Input: part model. Units: mm. Frame: model coordinates. Face numbers are marked on the shaded views. A direction names the side the tool comes from. Give positions to 0.01 mm unless a question says otherwise; leave off trailing zeros. Loops run counter-clockwise (first coordinate to the right, second up) from the corner with the lowest first, then second, coordinate; pieces in that order, holes last. Notation, with made-up numbers: (66.25, -14.75) -> (74.25, -14.75) arc R14 cw to (74.25, 8.25) -> close; hole circle Ø2 at (7, 1). An arc over 180 degrees is marked (long way). Answer as a JSON object with one key per item and string values. Group by question number.
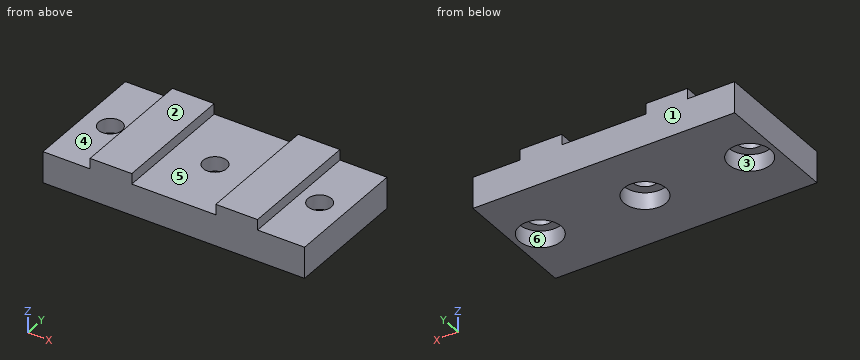
```python
from build123d import *

# Parameters (mm, degrees)
SKETCH1_W          = 39.6748
SKETCH1_H          = 19.05
EXTRUDE1_DEPTH     = 6.35
SKETCH2_W          = 7.1374
SKETCH2_H          = 1.6002
SKETCH2_W_2        = 12.7508
CUT_EXTRUDE1_DEPTH = 20.05
HOLE1_D            = 3.556
HOLE1_CBORE_D      = 6.35
HOLE1_CBORE_DEPTH  = 2.54


with BuildPart() as part:
    # Sketch1 → Extrude1 (new body)
    with BuildSketch(Plane.XY):
        with Locations((19.8374, 9.525)):
            Rectangle(SKETCH1_W, SKETCH1_H)
    extrude(amount=EXTRUDE1_DEPTH)

    # Sketch2 → Cut-Extrude1 (cut, through all)
    with BuildSketch(Plane.XZ):
        with Locations((3.5687, 5.5499)):
            Rectangle(SKETCH2_W, SKETCH2_H)
        with Locations((19.8374, 5.5499)):
            Rectangle(SKETCH2_W_2, SKETCH2_H)
        with Locations((36.1061, 5.5499)):
            Rectangle(SKETCH2_W, SKETCH2_H)
    extrude(amount=-CUT_EXTRUDE1_DEPTH, mode=Mode.SUBTRACT)

    # Hole1 (through all)
    with Locations(Plane(origin=(0, 0, 0), x_dir=(-1, 0, 0), z_dir=(0, 0, -1))):
        with Locations((-3.9624, 9.525), (-19.8374, 9.525), (-35.7124, 9.525)):
            CounterBoreHole(HOLE1_D / 2, HOLE1_CBORE_D / 2, HOLE1_CBORE_DEPTH)


solid = part.part
```
Q1. Ray query, probe 1 along X at (y, z) = (8.5, 3.75); probe 2 along Z at (x, y) = (26, 11.75); probe 3 along Y at (x, z) = (4, 0.5). Return the intervals inside material, ascending.
Q2. Section B-B on z = 4.25. Return the cut outline in (x, y) (3 decimals), then the cut area to 3 significant figures.
Q3. Section A-A on x = 35.5. Return the cut outline in (y, z), then the cut area to 3 significant figures.
Q4. Pull-direction query (Y, two-part tool) for the marked faces 1, 2 and 3; classes: +Y half, -Y half, draft (parallel to the pull), parting line (faces both ways), or undercut.
Q5. Section C-C on y = 2.75. Return the cut outline in (x, z), then the cut area to 3 significant figures.
Q6. Section D-D on x = 19.5. Return the cut outline in (y, z), then the cut area to 3 significant figures.
Q7. Set-up query: the marked faces 4, 5 and 6. Return all of +Z, -Z, +X, -X, +Y, -Y with unobstructed straight access to the full face (end or side cutting, diameter ignored); none if empty.
Q8. Pin query (flat end, axial travel): pin 1 Ø0.5 at (y, z) = (11.5, 5.5) entering from +X; pin 2 Ø5 at (x, y) = (18.5, 8.5) entering from -Z; pin 3 Ø4.5 at (x, y) = (3.96, 9.52) entering from +Z; pin 4 Ø3 at (x, y) = (19.84, 9.52) entering from +Z. Return the tip coordinate at first contact, or that it passes through.
Numbers:
{
 "1": {"probe 1": "x = 0 to 2.51, 5.42 to 18.38, 21.29 to 34.26, 37.17 to 39.67", "probe 2": "z = 0 to 4.75", "probe 3": "y = 0 to 6.35, 12.7 to 19.05"},
 "2": {"outline": "(0, 0) -> (39.675, 0) -> (39.675, 19.05) -> (0, 19.05) -> close; hole circle Ø3.556 at (3.962, 9.525); hole circle Ø3.556 at (19.837, 9.525); hole circle Ø3.556 at (35.712, 9.525)", "area": "726 mm²"},
 "3": {"outline": "(0, 0) -> (6.36, 0) -> (6.36, 2.54) -> (7.76, 2.54) -> (7.76, 4.75) -> (0, 4.75) -> close; (11.29, 2.54) -> (12.69, 2.54) -> (12.69, 0) -> (19.05, 0) -> (19.05, 4.75) -> (11.29, 4.75) -> close", "area": "66.6 mm²"},
 "4": {"face 1": "+Y half", "face 2": "draft", "face 3": "undercut"},
 "5": {"outline": "(0, 0) -> (39.67, 0) -> (39.67, 4.75) -> (32.54, 4.75) -> (32.54, 6.35) -> (26.21, 6.35) -> (26.21, 4.75) -> (13.46, 4.75) -> (13.46, 6.35) -> (7.14, 6.35) -> (7.14, 4.75) -> (0, 4.75) -> close", "area": "209 mm²"},
 "6": {"outline": "(0, 0) -> (6.37, 0) -> (6.37, 2.54) -> (7.78, 2.54) -> (7.78, 4.75) -> (0, 4.75) -> close; (11.27, 2.54) -> (12.68, 2.54) -> (12.68, 0) -> (19.05, 0) -> (19.05, 4.75) -> (11.27, 4.75) -> close", "area": "66.7 mm²"},
 "7": {"face 4": "+Z, -X, +Y, -Y", "face 5": "+Z, +Y, -Y", "face 6": "-Z"},
 "8": {"pin 1": "stops at x = 32.54", "pin 2": "stops at z = 0", "pin 3": "stops at z = 4.75", "pin 4": "passes through"}
}
